```python
from build123d import *

# Parameters (mm, degrees)
F0_R          = 25
F0_R_2        = 10
F1_DEPTH      = 15
F1_DEPTH_BACK = 15
F0_R_3        = 2
F2_DEPTH      = 10
F2_DEPTH_BACK = 10
F3_R          = 3


with BuildPart() as f1:
    # F0 (on Front) → F1 (new body, two sides)
    with BuildSketch(Plane.XZ) as f1_sk:
        Circle(F0_R)
        Circle(F0_R_2, mode=Mode.SUBTRACT)
    extrude(amount=F1_DEPTH)
    extrude(f1_sk.sketch, amount=-F1_DEPTH_BACK)

    # F0 (on Front) → F2 (join, two sides)
    with BuildSketch(Plane.XZ) as f2_sk:
        Circle(F0_R_2)
        Circle(F0_R_3, mode=Mode.SUBTRACT)
    extrude(amount=F2_DEPTH)
    extrude(f2_sk.sketch, amount=-F2_DEPTH_BACK)

    # F3
    f3_edges = [f1.edges().sort_by_distance(p)[0] for p in [
        (-25, 15, 0),
        (-25, -15, 0),
        (-10, -15, 0),
        (-10, 15, 0),
    ]]
    fillet(f3_edges, radius=F3_R)


solid = f1.part
```
Check sheet for the modelled part. Datum: model origin and axes. Units: mm. A direction names the side the tool comes from. Coordinates: 2 decimals unless noted, no trailing zeros. Loops run counter-clockwise (first coordinate to the right, second up) from the corner with the lowest first, then second, coordinate; pieces in that order, holes last.
1) Sectioned sample at C-C (y = 5). Record the boundary of the cut face in (x, z).
2) Gauge pin test, flat ends, axial feed: pin 1 (16 mm diameter, centred on x = -2, z = 3, fed in from -Y); pin 2 (6 mm diameter, centred on x = -14, y = -4, fed in from +Z); pin 3 (8 mm diameter, centred on x = -3.5, y = 6.5, fed in from -Z). Record the tip position at first contact, or that the pin passes through.
3) Sectioned sample at B-B (z = 0). Record the boundary of the cut face in (x, y).
4) Material ranges on probe 1 along Z at (x, y) = (0, -5); probe 2 along Z at (x, y) = (0, -11.25); probe 3 along Y at (x, z) = (-4, 3.5), recorded low to high.
5) Sectioned sample at A-A (x = 0). Record the boundary of the cut face in (y, z).
6) Release check for a two-part mould opening along Z. For faces 1 (the face through (9.5, 15, -9.5)), 2 (the face through (23.846, -0.168, 7.509)), 3 (the face through (-2.17, 10.99, -9.76)) record: released by +Z, released by -Z, zero draft, split by the parting line, or undercut.
7) Access from +Z, -Z, +X, -X, +Y, -Y to the whole of each face (thin tool, end or side, straight path). Record for faces 4 (the face through (-2.17, -10.99, -9.76)), 5 (the face through (9.5, -15, -9.5)), 6 (the face through (-0.1, 10, 2.4)).
Check sheet entries:
1. outline: circle Ø50 at (0, 0); hole circle Ø4 at (0, 0)
2. pin 1: stops at y = -14.66
2. pin 2: stops at z = 22.45
2. pin 3: stops at z = -25
3. outline: (-25, -12) arc R3 ccw to (-22, -15) - (-13, -15) arc R3 ccw to (-10, -12) - (-10, -10) - (-2, -10) - (-2, 10) - (-10, 10) - (-10, 12) arc R3 ccw to (-13, 15) - (-22, 15) arc R3 ccw to (-25, 12) - close; (2, -10) - (10, -10) - (10, -12) arc R3 ccw to (13, -15) - (22, -15) arc R3 ccw to (25, -12) - (25, 12) arc R3 ccw to (22, 15) - (13, 15) arc R3 ccw to (10, 12) - (10, 10) - (2, 10) - close
4. probe 1: z = -25 to -2, 2 to 25
4. probe 2: z = -25 to -10, 10 to 25
4. probe 3: y = -10 to 10
5. outline: (-15, -22) arc R3 ccw to (-12, -25) - (12, -25) arc R3 ccw to (15, -22) - (15, -13) arc R3 ccw to (12, -10) - (10, -10) - (10, -2) - (-10, -2) - (-10, -10) - (-12, -10) arc R3 ccw to (-15, -13) - close; (-15, 13) arc R3 ccw to (-12, 10) - (-10, 10) - (-10, 2) - (10, 2) - (10, 10) - (12, 10) arc R3 ccw to (15, 13) - (15, 22) arc R3 ccw to (12, 25) - (-12, 25) arc R3 ccw to (-15, 22) - close
6. face 1: zero draft
6. face 2: split by the parting line
6. face 3: undercut
7. face 4: -Y
7. face 5: +Z, -Z, +X, -X, -Y
7. face 6: +Y
